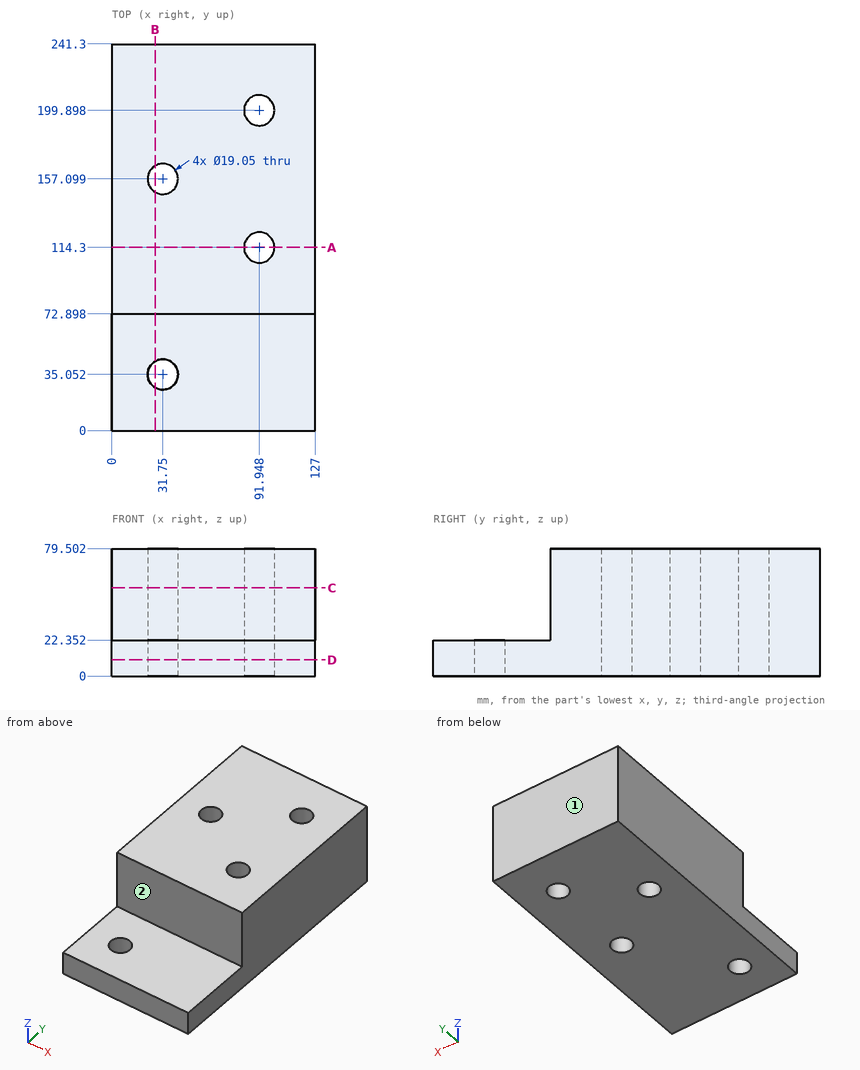
Check sheet for the drawn part. Datum: minimum x, y, z corner. Units: mm. A direction names the side the tool comes from. Round coordinates to 2 decimals unless told otherwise and drop trailing zeros. Order: outer loops, then holes, each group sorted by start corner. A loop starts at its lowest first (then second) coordinate and runs counter-clockwise, first axis right, second up. Notation, with made-up numbers: M 4.5,-29 L 54.5,-29 A16 cw 54.5,-12 Z; hole C 65,37.5 d6. An arc over 180 degrees is marked long. Answer in a Markdown table with one row per item.
(1) Section check B-B on x = 27. Record the boundary of the cut face in (y, z).
Findings:
| item | result |
|---|---|
| outline | M 0,0 L 26.8,0 L 26.8,22.35 L 0,22.35 Z; M 43.31,0 L 148.84,0 L 148.84,79.5 L 72.9,79.5 L 72.9,22.35 L 43.31,22.35 Z; M 165.36,0 L 241.3,0 L 241.3,79.5 L 165.36,79.5 Z |
(2) Material ranges on line 1 along Y through (x, z) = (31.75, 7.5); line 2 along Y through (x, z) = (31, 8); line 3 along Y through (x, z) = (31.75, 47.5), recorded low to high. Write a range as from..to.
Findings:
| item | result |
|---|---|
| line 1 | y = 0..25.53, 44.58..147.57, 166.62..241.3 |
| line 2 | y = 0..25.56, 44.55..147.6, 166.59..241.3 |
| line 3 | y = 72.9..147.57, 166.62..241.3 |
(3) Section check C-C on z = 55. Record the boundary of the cut face in (x, y) (3 decimals).
Findings:
| item | result |
|---|---|
| outline | M 0,72.898 L 127,72.898 L 127,241.3 L 0,241.3 Z; hole C 31.75,157.099 d19.05; hole C 91.948,114.3 d19.05; hole C 91.948,199.898 d19.05 |
(4) Gauge pin test, flat ends, axial feed: pin 1 (6 mm diameter, centred on y = 85.5, z = 66, fed in from -X); pin 2 (11.5 mm diameter, centred on x = 31.75, y = 35.052, fed in from -Z). Record the tip position at first contact, or that the pin passes through.
Findings:
| item | result |
|---|---|
| pin 1 | stops at x = 0 |
| pin 2 | passes through |
(5) Set-up check for the marked faces 1 and 2: record each of +Z, -Z, +X, -X, +Y, -Y from which the full face is reachable in a straight line by a thin tool's end or side.
Findings:
| item | result |
|---|---|
| face 1 | +Z, -Z, +X, -X, +Y |
| face 2 | +Z, +X, -X, -Y |
(6) Section check A-A on y = 114.3. Record the boundary of the cut face in (x, z).
Findings:
| item | result |
|---|---|
| outline | M 0,0 L 82.42,0 L 82.42,79.5 L 0,79.5 Z; M 101.47,0 L 127,0 L 127,79.5 L 101.47,79.5 Z |
(7) Section check D-D on z = 10. Record the boundary of the cut face in (x, y) (3 decimals), plus the area to 3 significant figures.
Findings:
| item | result |
|---|---|
| outline | M 0,0 L 127,0 L 127,241.3 L 0,241.3 Z; hole C 31.75,35.052 d19.05; hole C 31.75,157.099 d19.05; hole C 91.948,114.3 d19.05; hole C 91.948,199.898 d19.05 |
| area | 29,500 mm^2 |
